from build123d import *

# Parameters (mm, degrees)
SKETCH3_R           = 10
BOSS_EXTRUDE1_DEPTH = 3


with BuildPart() as part:
    # Sketch1 → Revolve1 (revolve)
    with BuildSketch(Plane.XY, mode=Mode.PRIVATE) as revolve1_sk:
        Polygon((0, 0), (0, 130), (6, 130), (6, 122.525384953), (6, 0), align=None)
    revolve(revolve1_sk.sketch.rotate(Axis((0, 0, 0), (0, 1, 0)), 90), axis=Axis((0, 0, 0), (0, 1, 0)))

    # Sketch2 → Revolve2 (revolve)
    with BuildSketch(Plane.XY, mode=Mode.PRIVATE) as revolve2_sk:
        Polygon((0, 130), (18, 130), (18, 126.185810056), (16.418354863, 125), (18, 123.913651393), (18, 120), (0, 120), align=None)
    revolve(revolve2_sk.sketch.rotate(Axis((0, 130, 0), (0, -1, 0)), 180), axis=Axis((0, 130, 0), (0, -1, 0)))

    # Sketch3 → Boss-Extrude1 (add)
    with BuildSketch(Plane.XZ):
        with Locations(Location((0, 0, 0), (0, 0, 270))):
            Circle(SKETCH3_R)
    extrude(amount=BOSS_EXTRUDE1_DEPTH)


solid = part.part
Read the model definition and answer for the solid it produces. Units are mm, in the model's axes. A direction names the side the tool comes from. Coordinates: 2 decimals unless noted, no trailing zeros. Loops run counter-clockwise (first coordinate to the right, second up) from the corner with the lowest first, then second, coordinate; pieces in that order, holes last. Notation, with made-up numbers: (82, 82.25) - (134, 82.25) arc R13 ccw to (134, 103.25) - close; hole circle Ø11 at (29.25, 3). An arc over 180 degrees is marked (long way). Answer in a Markdown table with one row per item.
Q1. Find section C-C on y = 94.5. Write down the section's boundary in (x, z), plus the area to 3 significant figures.
Here are the results:
| item | result |
|---|---|
| outline | circle Ø12 at (0, 0) |
| area | 113 mm^2 |
Q2. Find section A-A on z = 0. Write down the section's boundary in (x, y).
Here are the results:
| item | result |
|---|---|
| outline | (-18, 120) - (-6, 120) - (-6, 0) - (-10, 0) - (-10, -3) - (10, -3) - (10, 0) - (6, 0) - (6, 120) - (18, 120) - (18, 123.91) - (16.42, 125) - (18, 126.19) - (18, 130) - (-18, 130) - (-18, 126.19) - (-16.42, 125) - (-18, 123.91) - close |
Q3. Given P1, Ø1.5, axis at x = 5.5, z = 13, coming from the -Y side; P2, Ø6, axis at x = -7, y = 51.5, coming from the +Z side, each flat-ended and moving along its own axis, determine where each tip first touches the part or whether it passes through.
Here are the results:
| item | result |
|---|---|
| P1 | stops at y = 120 |
| P2 | stops at z = 4.47 |
Q4. Find section B-B on x = 0. Write down the section's boundary in (y, z).
Here are the results:
| item | result |
|---|---|
| outline | (-3, -10) - (0, -10) - (0, -6) - (120, -6) - (120, -18) - (123.91, -18) - (125, -16.42) - (126.19, -18) - (130, -18) - (130, 18) - (126.19, 18) - (125, 16.42) - (123.91, 18) - (120, 18) - (120, 6) - (0, 6) - (0, 10) - (-3, 10) - close |
Q5. Straight lines are drawn through the part: line 1 along Y through (x, z) = (8, 5); line 2 along Y through (x, z) = (12.5, 9); line 3 along Y through (x, z) = (15.5, -6.5). For each, find the intervals that lie inside material, in ascending order. Write a range as [from, to].
Here are the results:
| item | result |
|---|---|
| line 1 | y = [-3, 0], [120, 130] |
| line 2 | y = [120, 130] |
| line 3 | y = [120, 124.73], [125.29, 130] |
Q6. For faces 1 (the cylindrical face through (-1.802, 60.84, -5.723)), 2 (the cylindrical face through (13.267, 121.929, -12.165)), determine the directions among +Z, -Z, +X, -X, +Y, -Y from which every point of the face is accessible in a straight line to the end or side of a thin tool.
Here are the results:
| item | result |
|---|---|
| face 1 | none |
| face 2 | +Y, -Y |
Q7. The mould has two halves that part along Y. Classify faces 3 (the flat face through (0, 120, 8)), 4 (the flat face through (0, -3, 0)), 5 (the cylindrical face through (-9.76, -1.48, 2.17)): pulls with the +Y half, pulls with the -Y half, needs draft (parallel to the pull), parting line crosses it, or undercut.
Here are the results:
| item | result |
|---|---|
| face 3 | undercut |
| face 4 | pulls with the -Y half |
| face 5 | needs draft |
